```python
from build123d import *

# Parameters (mm, degrees)
BOSS_EXTRUDE1_DEPTH     = 15.045877519
BOSS_EXTRUDE2_DEPTH     = 30
BOSS_EXTRUDE3_DEPTH     = 160
CUT_EXTRUDE1_DEPTH      = 397.42670329
CUT_EXTRUDE1_DEPTH_BACK = 397.42670329
SKETCH5_W               = 30
SKETCH5_H               = 30
CUT_EXTRUDE2_START      = -30
CUT_EXTRUDE2_DEPTH      = 30
CUT_EXTRUDE3_DEPTH      = 2.010455065
BOSS_EXTRUDE6_START     = -34.448076
BOSS_EXTRUDE6_DEPTH     = 68.896152
SKETCH13_W              = 15
SKETCH13_H              = 30
BOSS_EXTRUDE7_DEPTH     = 10
SKETCH14_W              = 15
SKETCH14_H              = 30
BOSS_EXTRUDE8_DEPTH     = 10
CUT_EXTRUDE6_DEPTH      = 192
SKETCH18_R              = 3
CUT_EXTRUDE7_DEPTH      = 192
CUT_EXTRUDE8_REACH      = 232.854
SKETCH19_R              = 5.5
FILLET2_R               = 2.5


# Read off the part's stored shape, not the designer's step: Boss-Extrude3
with BuildPart() as part:
    # Sketch1 → Boss-Extrude1 (new body)
    with BuildSketch(Plane(origin=(0, 0, 0), x_dir=(1, 0, 0), z_dir=(0, 1, 0))):
        with BuildLine():
            Line((-185, -65), (5, -65))
            ThreePointArc((5, -65), (60.514401442, -84.704810384), (91.182336182, -135))
            Line((91.182336182, -135), (185, -135))
            Line((185, -135), (185, 135))
            Line((185, 135), (-185, 135))
            Line((-185, 135), (-185, -65))
        make_face()
    extrude(amount=BOSS_EXTRUDE1_DEPTH)

    # Sketch2 → Boss-Extrude2 (add)
    with BuildSketch(Plane(origin=(0, 15.045877519, 0), x_dir=(1, 0, 0), z_dir=(0, 1, 0))):
        Polygon((-175, -35), (-175, 30), (-185, 30), (-185, -45), (-142.5, -45), (-142.5, -35), align=None)
        Polygon((-175, 125), (-142.5, 125), (-142.5, 135), (-185, 135), (-185, 60), (-175, 60), align=None)
        Polygon((-95, -35), (-95, 30), (-85, 30), (-85, -45), (-127.5, -45), (-127.5, -35), align=None)
        Polygon((-127.5, 135), (-127.5, 125), (-95, 125), (-95, 60), (-85, 60), (-85, 135), align=None)
    extrude(amount=BOSS_EXTRUDE2_DEPTH)

    # Boss-Extrude3 outline → Boss-Extrude3 (add)
    with BuildSketch(Plane.XY.offset(-125)):
        with BuildLine():
            ThreePointArc((-95, 45.045877519), (-110, 23.379210852), (-135, 15.045877519))
            Line((-135, 15.045877519), (-95, 15.045877519))
            Line((-95, 15.045877519), (-95, 45.045877519))
        make_face()
        with BuildLine():
            Line((-175, 45.045877519), (-175, 15.045877519))
            Line((-175, 15.045877519), (-135, 15.045877519))
            ThreePointArc((-135, 15.045877519), (-160, 23.379210852), (-175, 45.045877519))
        make_face()
    extrude(amount=BOSS_EXTRUDE3_DEPTH)

    # Sketch5 → Cut-Extrude1 (cut, two sides: drawn at the far end of the back side and taken through both)
    with BuildSketch(Plane.ZY.offset(185).offset(-CUT_EXTRUDE1_DEPTH_BACK)):
        with Locations((-45, 30.045877519)):
            Rectangle(SKETCH5_W, SKETCH5_H)
    extrude(amount=CUT_EXTRUDE1_DEPTH + CUT_EXTRUDE1_DEPTH_BACK, mode=Mode.SUBTRACT)

    # Sketch6 → Cut-Extrude2 (cut)
    with BuildSketch(Plane(origin=(0, 15.045877519, 0), x_dir=(1, 0, 0), z_dir=(0, 1, 0)).offset(CUT_EXTRUDE2_START)):
        with BuildLine():
            Line((-85, 135), (-85, 60))
            Line((-85, 60), (-85, 30))
            Line((-85, 30), (-85, -45))
            Line((-85, -45), (-127.5, -45))
            Line((-127.5, -45), (-142.5, -45))
            Line((-142.5, -45), (-185, -45))
            Line((-185, -45), (-185, -65))
            Line((-185, -65), (5, -65))
            ThreePointArc((5, -65), (60.514401442, -84.704810384), (91.182336182, -135))
            Line((91.182336182, -135), (185, -135))
            Line((185, -135), (185, 135))
            Line((185, 135), (-85, 135))
        make_face()
    extrude(amount=CUT_EXTRUDE2_DEPTH, mode=Mode.SUBTRACT)

    # Sketch8 → Cut-Extrude3 (cut)
    with BuildSketch(Plane(origin=(0, 15.045877519, 0), x_dir=(1, 0, 0), z_dir=(0, 1, 0))):
        Polygon((-135, 60), (-185, 60), (-185, 30), (-135, 30), (-85, 30), (-85, 60), align=None)
    extrude(amount=-CUT_EXTRUDE3_DEPTH, mode=Mode.SUBTRACT)

    # Sketch12 → Boss-Extrude6 (add)
    with BuildSketch(Plane(origin=(-135, 0, 0), x_dir=(0, 0, -1), z_dir=(1, 0, 0)).offset(BOSS_EXTRUDE6_START)):
        with BuildLine():
            Line((-35, 33.272382456), (-35, 15.00790917))
            Line((-35, 15.00790917), (30, 15.045877519))
            add(Edge.make_bspline(
                [(-35, 33.272382456), (-23.622698209, 24.45769668), (30, 15.045877519)],
                knots=[0, 0, 0, 1, 1, 1], degree=2))
        make_face()
    boss_extrude6 = extrude(amount=BOSS_EXTRUDE6_DEPTH)

    # Sketch13 → Boss-Extrude7 (add)
    with BuildSketch(Plane.XY.offset(45)):
        with Locations((-135, 30.045877519)):
            Rectangle(SKETCH13_W, SKETCH13_H)
    extrude(amount=-BOSS_EXTRUDE7_DEPTH)

    # Sketch14 → Boss-Extrude8 (add)
    with BuildSketch(Plane(origin=(0, 0, -135), x_dir=(-1, 0, 0), z_dir=(0, 0, -1))):
        with Locations((135, 30.045877519)):
            Rectangle(SKETCH14_W, SKETCH14_H)
    extrude(amount=-BOSS_EXTRUDE8_DEPTH)

    # Mirror3: Boss-Extrude6 across plane
    add(boss_extrude6.mirror(Plane.XY.offset(-45)))

    # Sketch9 → Cut-Extrude6 (cut)
    with BuildSketch(Plane.XY.offset(45)):
        with BuildLine():
            Line((-150, 45.045877519), (-120, 45.045877519))
            ThreePointArc((-120, 45.045877519), (-121.500780237, 34.041891851), (-125.767198961, 23.788223571))
            Line((-125.767198961, 23.788223571), (-144.232801039, 23.788223571))
            ThreePointArc((-144.232801039, 23.788223571), (-148.499219763, 34.041891851), (-150, 45.045877519))
        make_face()
    extrude(amount=-CUT_EXTRUDE6_DEPTH, mode=Mode.SUBTRACT)

    # Sketch18 → Cut-Extrude7 (cut)
    with BuildSketch(Plane.XZ):
        with Locations(Location((-135, 28.073614807, 0), (0, 0, 270))):
            Circle(SKETCH18_R)
    cut_extrude7 = extrude(amount=-CUT_EXTRUDE7_DEPTH, mode=Mode.SUBTRACT)

    # Sketch19 → Cut-Extrude8 (cut, up to next)
    with BuildSketch(Plane(origin=(0, 16, 0), x_dir=(-1, 0, 0), z_dir=(0, -1, 0)), mode=Mode.PRIVATE) as cut_extrude8_sk1:
        with Locations(Location((135, -28.073614807, 0), (0, 0, 90))):
            Circle(SKETCH19_R)
    cut_extrude8_tool1 = extrude(cut_extrude8_sk1.sketch, amount=-CUT_EXTRUDE8_REACH, mode=Mode.PRIVATE) & part.part
    cut_extrude8 = cut_extrude8_tool1.solids().sort_by_distance((-135, 16, 28.073615))[0]
    add(cut_extrude8, mode=Mode.SUBTRACT)

    # Mirror4: Cut-Extrude7, Cut-Extrude8 across plane
    add(cut_extrude7.mirror(Plane.XY.offset(-45)), mode=Mode.SUBTRACT)
    add(cut_extrude8.mirror(Plane.XY.offset(-45)), mode=Mode.SUBTRACT)

    # Fillet2
    fillet2_edges = [part.edges().sort_by_distance(p)[0] for p in [
        (-85, 13.035422455, -45),
        (-185, 13.035422455, -45),
        (-185, 29.040649987, -30),
        (-185, 29.040649987, -60),
        (-85, 29.040649987, -60),
        (-85, 29.040649987, -30),
    ]]
    fillet(fillet2_edges, radius=FILLET2_R)


solid = part.part
```
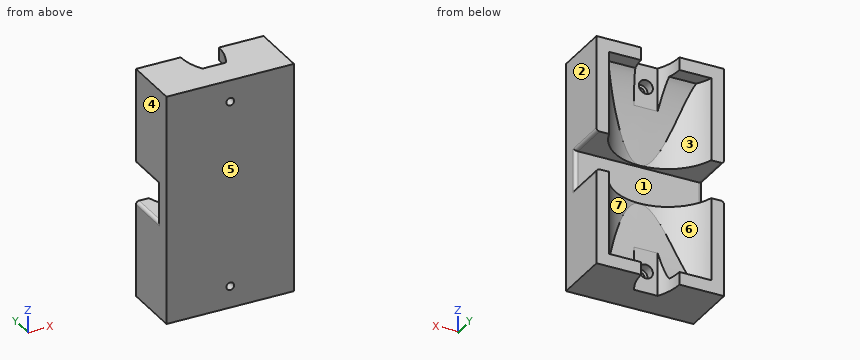
Model file for the job. Use its own axes, mm. Face numbers are marked on the shaded views. A direction names the side the tool comes from. Round coordinates to 2 decimals unless told otherwise and drop trailing zeros. Use CSV: the item, a comma, the result in double quotes. Start each with the question number.
Item 1: Pin check, flat tips, straight feed: P1, Ø4, axis at x = -160.5, z = -27, coming from the +Y side; P2, Ø10, axis at x = -135, z = 28.07, coming from the +Y side; P3, Ø9, axis at x = -139, z = 31.5, coming from the +Y side. Stop position of each tip, or through.
Item 2: Drill centre lines: L1, parallel to Z at x = -135, y = 7; L2, parallel to Z at x = -159.5, y = 14; L3, parallel to X at y = 24, z = -87.5. Where is each one in solid material? Low to high. Write a range as [from, to].
Item 3: Tool access for the marked faces 1, 2 and 3: list every direction of +Z, -Z, +X, -X, +Y, -Y with a clear straight run to the whole face (end or side of a thin tool).
Item 4: Two-plate mould, pull along X, no slides. Class the marked faces 4, 5, 6 and 7: released by +X, released by -X, zero draft, split by the parting line, or undercut.
Checked values:
1,P1,"stops at y = 25.41"
1,P2,"stops at y = 16"
1,P3,"stops at y = 23.79"
2,L1,"z = [-135, -121.07], [-115.07, 25.07], [31.07, 45]"
2,L2,"z = [-135, -60], [-30, 45]"
2,L3,"x = [-185, -160.81], [-109.19, -85]"
3,face 1,"+X, -X, +Y"
3,face 2,"+Z, -Z, +X, +Y, -Y"
3,face 3,"+Y"
4,face 4,"released by -X"
4,face 5,"zero draft"
4,face 6,"undercut"
4,face 7,"undercut"
